from build123d import *

# Parameters (mm, degrees)
F0_R     = 29.75
F2_DEPTH = 3.15
F1_W     = 5.5
F1_H     = 24.426396
F3_DEPTH = 3.15
F4_R     = 3


with BuildPart() as f2:
    # F0 (on Top) → F2 (new body)
    with BuildSketch(Plane.XY):
        Circle(F0_R)
    extrude(amount=F2_DEPTH)

    # F1 (on Top) → F3 (cut)
    with BuildSketch(Plane.XY):
        Rectangle(F1_W, F1_H)
    extrude(amount=F3_DEPTH, mode=Mode.SUBTRACT)

    # F4
    f4_edges = [f2.edges().sort_by_distance(p)[0] for p in [
        (-29.75, 0, 0),
    ]]
    fillet(f4_edges, radius=F4_R)


solid = f2.part
Geometry: final body of the model. Coordinates: model frame, mm. A direction names the side the tool comes from. Round coordinates to 2 decimals unless told otherwise and drop trailing zeros. Order: outer loops, then holes, each group sorted by start corner. A loop starts at its lowest first (then second) coordinate and runs counter-clockwise, first axis right, second up.
Q1. Section A-A, the plane y = 0. Output: boundary loops of the cut face in (x, z).
Result sheet:
outline: (-29.75, 3) arc R3 ccw to (-26.75, 0) - (-2.75, 0) - (-2.75, 3.15) - (-29.75, 3.15) - close; (2.75, 0) - (26.75, 0) arc R3 ccw to (29.75, 3) - (29.75, 3.15) - (2.75, 3.15) - close
Q2. Mould query, pull axis X, two halves, no side actions, for faces 1 (the face through (0, -12.213, 2)), 2 (the face through (6, 0, 3.15)). Classes: released by +X, released by -X, zero draft, split by the parting line, or undercut.
Result sheet:
face 1: undercut
face 2: zero draft
Q3. Access query for faces 3 (the face through (-2.75, 0, 2)), 4 (the face through (6, 0, 0)). Directions: +Z, -Z, +X, -X, +Y, -Y. A direction counts if a zero-diameter tool reaches every point of the face in a straight line with its end or side. Return the directions, or none.
Result sheet:
face 3: +Z, -Z
face 4: -Z, +X, -X, +Y, -Y
Q4. Material intervals for probe 1 along X at (y, z) = (6, 0.3); probe 2 along X at (y, z) = (6.5, 2.5); probe 3 along Y at (x, z) = (-1, 0.95), sorted ascending.
Result sheet:
probe 1: x = -27.41 to -2.75, 2.75 to 27.41
probe 2: x = -28.99 to -2.75, 2.75 to 28.99
probe 3: y = -28.92 to -12.21, 12.21 to 28.92
Q5. Section B-B, the plane x = 0. Output: boundary loops of the cut face in (y, z).
Result sheet:
outline: (-29.75, 3) arc R3 ccw to (-26.75, 0) - (-12.21, 0) - (-12.21, 3.15) - (-29.75, 3.15) - close; (12.21, 0) - (26.75, 0) arc R3 ccw to (29.75, 3) - (29.75, 3.15) - (12.21, 3.15) - close
Q6. Section C-C, the plane z = 2.4. Output: boundary loops of the cut face in (x, y).
Result sheet:
outline: circle Ø59.38 at (0, 0); hole (-2.75, -12.21) - (2.75, -12.21) - (2.75, 12.21) - (-2.75, 12.21) - close
Q7. Pin query (flat end, axial travel): pin 1 (1 mm diameter, centred on x = -2.5, z = 2.5, fed in from -Y); pin 2 (1 mm diameter, centred on y = 17.5, z = 0.5, fed in from +X); pin 3 (1.6 mm diameter, centred on y = -3.5, z = 1.5, fed in from -X). Return the tip coordinate at first contact, or that it passes through.
Result sheet:
pin 1: stops at y = -29.67
pin 2: stops at x = 23.22
pin 3: stops at x = -29.48
